Design review of the part built by this model. Coordinates are the model's own, in mm. A direction names the side the tool comes from. Coordinates: 2 decimals unless noted, no trailing zeros. Loops run counter-clockwise (first coordinate to the right, second up) from the corner with the lowest first, then second, coordinate; pieces in that order, holes last. Notation, with made-up numbers: (53.25, -25.5) - (87.25, -25.5) arc R10 cw to (87.25, -17.5) - close; hole circle Ø11 at (-24, 25.5). An arc over 180 degrees is marked (long way). Return JSON: item names as keys, results as strings. Group by question number.
from build123d import *

# Parameters (mm, degrees)
SKETCH_W             = 42.762054
SKETCH_H             = 25.790352
PAD_DEPTH            = 5
PAD001_DEPTH         = 41
FILLET_R             = 10.85
FILLET001_R          = 10
SKETCH002_R          = 2.036707
POCKET_DEPTH         = 5.001
CHAMFER_SIZE         = 1
POCKET001_DEPTH      = 22
FILLET002_R          = 3
SKETCH004_R          = 10.7777
SKETCH004_R_2        = 4.77159
PAD002_DEPTH         = 5
PAD003_DEPTH         = 5
SKETCH006_R          = 4.840276
POCKET002_DEPTH      = 25.653292
POCKET002_DEPTH_BACK = -5.13906


with BuildPart() as part:
    # Sketch → Pad (new body)
    with BuildSketch(Plane.XY):
        Rectangle(SKETCH_W, SKETCH_H)
    extrude(amount=PAD_DEPTH)

    # Sketch001 (on Face6 of Pad) → Pad001 (join)
    with BuildSketch(Plane.XY.offset(5)):
        Polygon((-3.907949, -12.839293), (-3.907949, 8.895021), (-10.893314, 8.904404), (-10.893314, 12.757116), (10.893314, 12.757116), (10.893314, 8.812844), (3.240797, 8.812844), (3.240797, -12.839293), align=None)
    extrude(amount=PAD001_DEPTH)

    # Fillet
    fillet_edges = [part.edges().sort_by_distance(p)[0] for p in [
        (10.893314, 10.78498, 46),
        (-10.893314, 10.83076, 46),
    ]]
    fillet(fillet_edges, radius=FILLET_R)

    # Fillet001
    fillet001_edges = [part.edges().sort_by_distance(p)[0] for p in [
        (-10.893314, 10.83076, 5),
        (10.893314, 10.78498, 5),
    ]]
    fillet(fillet001_edges, radius=FILLET001_R)

    # Sketch002 (on Face1 of Fillet001) → Pocket (cut, through all)
    with BuildSketch(Plane.XY.offset(5)):
        with Locations((-15.012179, -7.460228)):
            Circle(SKETCH002_R)
        with Locations((15.012179, -7.460228)):
            Circle(SKETCH002_R)
    extrude(amount=-POCKET_DEPTH, mode=Mode.SUBTRACT)

    # Chamfer
    chamfer_edges = [part.edges().sort_by_distance(p)[0] for p in [
        (12.975472, -7.460228, 5),
        (-17.048886, -7.460228, 5),
    ]]
    chamfer(chamfer_edges, length=CHAMFER_SIZE)

    # Sketch003 (on Face12 of Chamfer) → Pocket001 (cut)
    with BuildSketch(Plane.YZ.offset(3.240797)):
        Polygon((8.830447, 27.110086), (-15.870471, 1.811423), (-31.901745, 27.110086), (-35.434662, 50.068335), (8.830447, 52.205082), align=None)
    extrude(amount=-POCKET001_DEPTH, mode=Mode.SUBTRACT)

    # Fillet002
    fillet002_edges = [part.edges().sort_by_distance(p)[0] for p in [
        (21.381027, -12.895176, 2.5),
        (-21.381027, -12.895176, 2.5),
    ]]
    fillet(fillet002_edges, radius=FILLET002_R)

    # Sketch004 (on Face16 of Fillet002) → Pad002 (join)
    with BuildSketch(Plane(origin=(0, 12.757116, 0), x_dir=(-1, 0, 0), z_dir=(0, 1, 0))):
        with Locations((0, 35.262314)):
            Circle(SKETCH004_R)
        with Locations((0, 35.262314)):
            Circle(SKETCH004_R_2, mode=Mode.SUBTRACT)
    extrude(amount=PAD002_DEPTH)

    # Sketch005 (on Face4 of Pad002) → Pad003 (join)
    with BuildSketch(Plane(origin=(0, 12.895176, 0), x_dir=(-1, 0, 0), z_dir=(0, 1, 0))):
        Polygon((-21.338758, 0.045037), (-21.338758, 2.59236), (21.34976, 2.59236), (21.34976, -0.041886), align=None)
    extrude(amount=PAD003_DEPTH)

    # Sketch006 (on Face40 of Pad003) → Pocket002 (cut, two sides)
    with BuildSketch(Plane(origin=(0, 12.757116, 0), x_dir=(-1, 0, 0), z_dir=(0, 1, 0))) as pocket002_sk:
        with Locations((0, 35.328526)):
            Circle(SKETCH006_R)
    extrude(amount=-POCKET002_DEPTH, mode=Mode.SUBTRACT)
    extrude(pocket002_sk.sketch, amount=-POCKET002_DEPTH_BACK, mode=Mode.SUBTRACT)


solid = part.part
Item 1: To check wall thickness, follow line 1 (Z direction, x = 0, y = 11); line 2 (X direction, y = 2, z = 10); line 3 (Z direction, x = -18, y = 15). State the ranges of each line that lie inside material, in increasing order. Write a range as from..to.
Item 2: Add section C-C (z = 26). State the section outline as (x, y) points, then the cut area to 3 significant figures.
Item 3: Add section A-A (z = 18). State the section outline as (x, y) points.
Item 4: For faces 4 (the face through (0, 15, 2.592)), 5 (the face through (-5, 17.757, 33)), 6 (the face through (-3.908, 3, 12)), 7 (the face through (10.893, 11, 25)), 8 (the face through (-21.381, 1, 2)), list the 3-axis set-ups (+Z, -Z, +X, -X, +Y, -Y) from which the entire face can be reached by the end or side of a thin tool; tool diameter is ignored.
Item 5: Add section B-B (y = 2). State the section outline as (x, z) points, then the cut area to 3 significant figures.
Item 6: Draft analysis for pull direction X (two halves, no side actions). For faces 1 (the face through (21.339, 15, 1)), 2 (the face through (-5, 0, 5)), 3 (the face through (-17.047, -7.371, 2.028)), state which applies: pulls with the +X half, pulls with the -X half, needs draft (parallel to the pull), parting line crosses it, or undercut.
Item 7: For P1, Ø1.3, axis at x = 2, z = 45.5, coming from the -Y side; P2, Ø5, axis at x = -3, y = -6.5, coming from the +Z side; P3, Ø3, axis at x = -7, y = -2.5, coming from the +Z side, all flat-tipped, find the tip position at first contact; note any pin that passes through.
Answers below:
{
 "1": {"line 1": "z = 0..30.49, 40.17..46", "line 2": "x = -3.91..3.24", "line 3": "z = -0.04..2.59"},
 "2": {"outline": "(-10.89, 8.9) - (-3.91, 8.9) - (-3.91, 7.75) - (3.24, 7.75) - (3.24, 8.81) - (10.89, 8.81) - (10.89, 12.76) - (5.51, 12.76) - (5.51, 17.76) - (-5.51, 17.76) - (-5.51, 12.76) - (-10.89, 12.76) - close", "area": "148 mm^2"},
 "3": {"outline": "(-10.89, 8.9) - (-3.91, 8.9) - (-3.91, -0.06) - (3.24, -0.06) - (3.24, 8.81) - (10.89, 8.81) - (10.89, 12.76) - (-10.89, 12.76) - close"},
 "4": {"face 4": "+X, -X, +Y", "face 5": "+Z, +X, -X, +Y", "face 6": "+Z, -X, -Y", "face 7": "+Z, +X, +Y, -Y", "face 8": "+Z, -Z, -X, +Y, -Y"},
 "5": {"outline": "(-21.38, 0) - (21.38, 0) - (21.38, 5) - (3.24, 5) - (3.24, 20.11) - (-3.91, 20.11) - (-3.91, 5) - (-21.38, 5) - close", "area": "322 mm^2"},
 "6": {"face 1": "pulls with the +X half", "face 2": "needs draft", "face 3": "undercut"},
 "7": {"P1": "stops at y = 8.83", "P2": "stops at z = 13.97", "P3": "stops at z = 5"}
}
